Design review of the part shown in the three views and the two pictorial views. Dimensions are in mm from the part's minimum x, y and z. Coordinates: 2 decimals unless noted, no trailing zeros. Loops run counter-clockwise (first coordinate to the right, second up) from the corner with the lowest first, then second, coordinate; pieces in that order, holes last. Notation, with made-up numbers: M 23.25,34 L 50.25,34 A21 ccw 50.25,65 Z; hole C -30,76.5 d8. An arc over 180 degrees is marked long. Answer as a JSON object with one key per item and string values. Group by question number.
Item 1: Add section B-B (z = 25). State the section outline as (x, y) points, then the cut area to 3 significant figures.
Item 2: Add section A-A (x = 35). State the section outline as (y, z) points.
Item 3: Add section C-C (y = 1.35). Count the separate pieces of the cut face and the enclosed holes in it, then the cut area to 3 significant figures.
Item 4: Wall thickness on L1, parallel to X at y = 1.2, z = 5; L2, parallel to Z at x = 30, y = 0.65; L3, parallel to X at y = 0.6, z = 35: over which ranges is each line inside the solid? List them lowest first. Write a range as from..to.
Item 5: Insertion check: pin 1 (12 mm diameter, centred on x = 42, z = 21.5, fed in from +Y); pin 2 (2.5 mm diameter, centred on x = 5, z = 5, fed in from -Y); pin 3 (0.8 mm diameter, centred on y = 1, z = 31.5, fed in from +X); pin 4 (0.8 mm diameter, centred on y = 1, z = 20.5, fed in from -X). Each pin has a flat end and moves straight along its axis. Give the tip position at first contact, or say it passes through.
Item 6: Add section D-D (z = 5). State the section outline as (x, y) points.
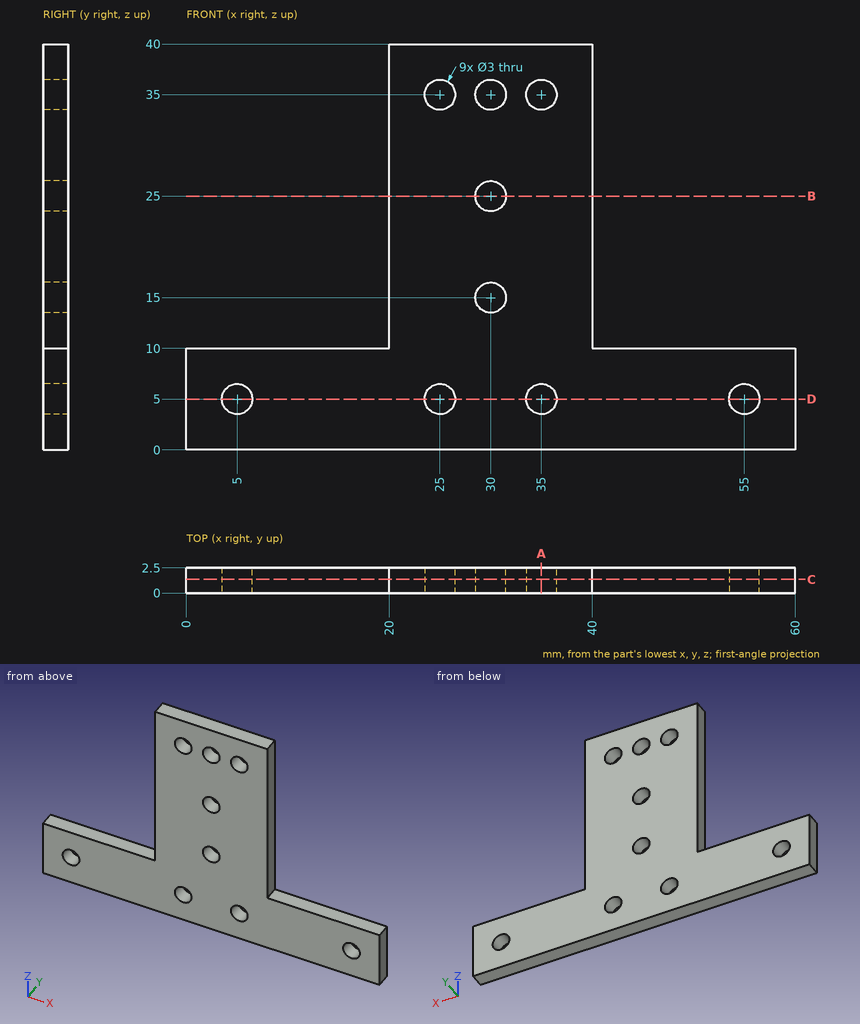
From the geometry:
{
 "1": {"outline": "M 20,0 L 28.5,0 L 28.5,2.5 L 20,2.5 Z; M 31.5,0 L 40,0 L 40,2.5 L 31.5,2.5 Z", "area": "42.5 mm²"},
 "2": {"outline": "M 0,0 L 2.5,0 L 2.5,3.5 L 0,3.5 Z; M 0,6.5 L 2.5,6.5 L 2.5,33.5 L 0,33.5 Z; M 0,36.5 L 2.5,36.5 L 2.5,40 L 0,40 Z"},
 "3": {"separate pieces": "1", "enclosed holes": "9", "area": "1,140 mm²"},
 "4": {"L1": "x = 0..3.5, 6.5..23.5, 26.5..33.5, 36.5..53.5, 56.5..60", "L2": "z = 0..13.5, 16.5..23.5, 26.5..33.5, 36.5..40", "L3": "x = 20..23.5, 26.5..28.5, 31.5..33.5, 36.5..40"},
 "5": {"pin 1": "stops at y = 2.5", "pin 2": "passes through", "pin 3": "stops at x = 40", "pin 4": "stops at x = 20"},
 "6": {"outline": "M 0,0 L 3.5,0 L 3.5,2.5 L 0,2.5 Z; M 6.5,0 L 23.5,0 L 23.5,2.5 L 6.5,2.5 Z; M 26.5,0 L 33.5,0 L 33.5,2.5 L 26.5,2.5 Z; M 36.5,0 L 53.5,0 L 53.5,2.5 L 36.5,2.5 Z; M 56.5,0 L 60,0 L 60,2.5 L 56.5,2.5 Z"}
}
